Design review of the part built by this model. Coordinates are the model's own, in mm. Give positions to 0.01 mm unless a question says otherwise; leave off trailing zeros. Write each loop counter-clockwise with the first axis right and the second up, starting at its lowest first coordinate (ties: lowest second). Pieces come first, ordered by that corner, then holes. Notation, with made-up numbers: M -13.75,-23.5 L -6.75,-23.5 A22 ccw -6.75,-10.5 Z; hole C 27.5,-36.5 d6. An arc over 180 degrees is marked long. Answer in a Markdown table with one row per item.
```python
from build123d import *

# Parameters (mm, degrees)
SKETCH1_R           = 6.82625
SKETCH1_R_2         = 4.445
BOSS_EXTRUDE1_DEPTH = 1.5875
SKETCH2_R           = 5.445
SKETCH2_R_2         = 4.445
EXTRUDE_THIN1_DEPTH = 1.5875
FILLET1_R           = 0.508


with BuildPart() as part:
    # Sketch1 → Boss-Extrude1 (new body)
    with BuildSketch(Plane.XY):
        with Locations((-6.731, -165.7192297)):
            Circle(SKETCH1_R)
        with Locations((-6.731, -165.7192297)):
            Circle(SKETCH1_R_2, mode=Mode.SUBTRACT)
    extrude(amount=BOSS_EXTRUDE1_DEPTH)

    # Sketch2 → Extrude-Thin1 (add)
    with BuildSketch(Plane.XY.offset(1.5875)):
        with Locations((-6.731, -165.7192297)):
            Circle(SKETCH2_R)
        with Locations((-6.731, -165.7192297)):
            Circle(SKETCH2_R_2, mode=Mode.SUBTRACT)
    extrude(amount=EXTRUDE_THIN1_DEPTH)

    # Fillet1
    fillet1_edges = [part.edges().sort_by_distance(p)[0] for p in [
        (-12.176, -165.7192297, 3.175),
        (-12.176, -165.7192297, 1.5875),
        (-13.55725, -165.7192297, 1.5875),
    ]]
    fillet(fillet1_edges, radius=FILLET1_R)


solid = part.part
```
1) Insertion check: P1, Ø4, axis at x = -7.5, y = -166, coming from the +Z side; P2, Ø1.5, axis at y = -166.5, z = 2, coming from the +X side; P3, Ø1.5, axis at y = -168, z = 0.5, coming from the -X side. Each pin has a flat end and moves straight along its axis. Give the tip position at first contact, or say it passes through.
Geometry says:
| item | result |
|---|---|
| P1 | through |
| P2 | x = 0.03 |
| P3 | x = -13.38 |
2) To check wall thickness, follow probe 1 along Z at (x, y) = (-8, -171.5); probe 2 along Y at (x, z) = (-3.25, 2.1); probe 3 along X at (y, z) = (-163.25, 2.5). State the ranges of each line that lie inside material, in increasing order. Write a range as [from, to].
Geometry says:
| item | result |
|---|---|
| probe 1 | [0, 1.59] |
| probe 2 | [-169.91, -168.48], [-162.96, -161.53] |
| probe 3 | [-11.58, -10.43], [-3.03, -1.88] |
3) The part is to be moulded in two halves that separate along X. For faces 1 (the face through (-7.911, -171.035, 2.377)), 2 (the face through (-9, -160, 1.588)), 3 (the face through (-7.31, -161.312, 1.565)), say which applies: released by +X, released by -X, zero draft, split by the parting line, or undercut.
Geometry says:
| item | result |
|---|---|
| face 1 | split by the parting line |
| face 2 | zero draft |
| face 3 | undercut |
4) Add section A-A (z = 2.4). Write out the cut boundary in (x, y) (3 decimals).
Geometry says:
| item | result |
|---|---|
| outline | C -6.731,-165.719 d10.89; hole C -6.731,-165.719 d8.89 |
5) Add section B-B (z = 0.4). Write out the cut boundary in (x, y) (1 decimal), and give its area (3 significant figures).
Geometry says:
| item | result |
|---|---|
| outline | C -6.7,-165.7 d13.7; hole C -6.7,-165.7 d8.9 |
| area | 84.3 mm^2 |
